Check sheet for the modelled part. Datum: model origin and axes. Units: mm. A direction names the side the tool comes from. Round coordinates to 2 decimals unless told otherwise and drop trailing zeros. Loops run counter-clockwise (first coordinate to the right, second up) from the corner with the lowest first, then second, coordinate; pieces in that order, holes last. Notation, with made-up numbers: (22.5, 40.5) -> (44.5, 40.5) arc R29 ccw to (44.5, 66.5) -> close; hole circle Ø5 at (-21, 70.25). An arc over 180 degrees is marked (long way). One line per question, with ' | ' between items.
```python
from build123d import *

# Parameters (mm, degrees)
SKETCH1_W           = 86.36
SKETCH1_H           = 50.8
SKETCH1_R           = 8.89
BOSS_EXTRUDE2_DEPTH = 25.4
CUT_EXTRUDE2_START  = 25.4
SKETCH1_3_R         = 13.97
SKETCH1_3_R_2       = 8.89
CUT_EXTRUDE2_DEPTH  = 5.08
CUT_EXTRUDE4_START  = -25.4
SKETCH1_4_R         = 13.97
SKETCH1_4_R_2       = 8.89
CUT_EXTRUDE4_DEPTH  = 5.08
SKETCH3_R           = 11.43
SKETCH3_R_2         = 5.55625
BOSS_EXTRUDE3_DEPTH = 10.16
SKETCH3_2_R         = 5.55625
CUT_EXTRUDE5_DEPTH  = 97.52
SKETCH4_W           = 66.04
SKETCH4_H           = 30.48
CUT_EXTRUDE6_DEPTH  = 51.8
BOSS_EXTRUDE4_START = 15.24
SKETCH5_R           = 17.78
SKETCH5_R_2         = 8.89
BOSS_EXTRUDE4_DEPTH = 5.08
BOSS_EXTRUDE5_START = -15.24
SKETCH5_2_R         = 17.78
SKETCH5_2_R_2       = 8.89
BOSS_EXTRUDE5_DEPTH = 5.08
FILLET1_R           = 2.54
FILLET2_R           = 2.54


with BuildPart() as part:
    # Sketch1 → Boss-Extrude2 (new body, symmetric)
    with BuildSketch(Plane.XY):
        Rectangle(SKETCH1_W, SKETCH1_H)
        Circle(SKETCH1_R, mode=Mode.SUBTRACT)
    extrude(amount=BOSS_EXTRUDE2_DEPTH, both=True)

    # Sketch1<3> → Cut-Extrude2 (cut)
    with BuildSketch(Plane.XY.offset(CUT_EXTRUDE2_START)):
        Circle(SKETCH1_3_R)
        Circle(SKETCH1_3_R_2, mode=Mode.SUBTRACT)
    extrude(amount=-CUT_EXTRUDE2_DEPTH, mode=Mode.SUBTRACT)

    # Sketch1<4> → Cut-Extrude4 (cut)
    with BuildSketch(Plane.XY.offset(CUT_EXTRUDE4_START)):
        Circle(SKETCH1_4_R)
        Circle(SKETCH1_4_R_2, mode=Mode.SUBTRACT)
    extrude(amount=CUT_EXTRUDE4_DEPTH, mode=Mode.SUBTRACT)

    # Sketch3 → Boss-Extrude3 (add)
    with BuildSketch(Plane(origin=(43.18, 0, 0), x_dir=(0, 0, -1), z_dir=(1, 0, 0))):
        Circle(SKETCH3_R)
        Circle(SKETCH3_R_2, mode=Mode.SUBTRACT)
    boss_extrude3 = extrude(amount=BOSS_EXTRUDE3_DEPTH)

    # Mirror1: Boss-Extrude3 across plane
    add(boss_extrude3.mirror(Plane(origin=(0, 0, 0), x_dir=(0, 0, 1), z_dir=(1, 0, 0))))

    # Sketch3<2> → Cut-Extrude5 (cut, through all)
    with BuildSketch(Plane(origin=(43.18, 0, 0), x_dir=(0, 0, -1), z_dir=(1, 0, 0))):
        Circle(SKETCH3_2_R)
    extrude(amount=-CUT_EXTRUDE5_DEPTH, mode=Mode.SUBTRACT)

    # Sketch4 → Cut-Extrude6 (cut, through all)
    with BuildSketch(Plane(origin=(0, 25.4, 0), x_dir=(1, 0, 0), z_dir=(0, 1, 0))):
        Rectangle(SKETCH4_W, SKETCH4_H)
    extrude(amount=-CUT_EXTRUDE6_DEPTH, mode=Mode.SUBTRACT)

    # Sketch5 → Boss-Extrude4 (add)
    with BuildSketch(Plane.XY.offset(BOSS_EXTRUDE4_START)):
        Circle(SKETCH5_R)
        Circle(SKETCH5_R_2, mode=Mode.SUBTRACT)
    extrude(amount=-BOSS_EXTRUDE4_DEPTH)

    # Sketch5<2> → Boss-Extrude5 (add)
    with BuildSketch(Plane.XY.offset(BOSS_EXTRUDE5_START)):
        Circle(SKETCH5_2_R)
        Circle(SKETCH5_2_R_2, mode=Mode.SUBTRACT)
    extrude(amount=BOSS_EXTRUDE5_DEPTH)

    # Fillet1
    fillet1_edges = [part.edges().sort_by_distance(p)[0] for p in [
        (-17.78, 0, 15.24),
        (-17.78, 0, -15.24),
    ]]
    fillet(fillet1_edges, radius=FILLET1_R)

    # Fillet2
    fillet2_edges = [part.edges().sort_by_distance(p)[0] for p in [
        (43.18, 0, 11.43),
        (-43.18, 0, 11.43),
    ]]
    fillet(fillet2_edges, radius=FILLET2_R)


solid = part.part
```
(1) Sectioned sample at A-A, the plane z = 0. Record the cut outline in (x, y).
Answer:
outline: (-53.34, -11.43) -> (-45.72, -11.43) arc R2.54 cw to (-43.18, -13.97) -> (-43.18, -25.4) -> (-33.02, -25.4) -> (-33.02, -5.56) -> (-53.34, -5.56) -> close; (-53.34, 5.56) -> (-33.02, 5.56) -> (-33.02, 25.4) -> (-43.18, 25.4) -> (-43.18, 13.97) arc R2.54 cw to (-45.72, 11.43) -> (-53.34, 11.43) -> close; (33.02, -25.4) -> (43.18, -25.4) -> (43.18, -13.97) arc R2.54 cw to (45.72, -11.43) -> (53.34, -11.43) -> (53.34, -5.56) -> (33.02, -5.56) -> close; (33.02, 5.56) -> (53.34, 5.56) -> (53.34, 11.43) -> (45.72, 11.43) arc R2.54 cw to (43.18, 13.97) -> (43.18, 25.4) -> (33.02, 25.4) -> close
(2) Go/stop test with flat-tipped pins: pin 1 (14 mm diameter, centred on x = 0.5, y = -4, fed in from -Z); pin 2 (1.5 mm diameter, centred on y = 9.5, z = -10.5, fed in from +X); pin 3 (5 mm diameter, centred on y = 14.5, z = 7, fed in from -X). Record where each tip stops, or that it passes through.
Answer:
pin 1: stops at z = -20.32 | pin 2: stops at x = 43.24 | pin 3: stops at x = -43.21
(3) Sectioned sample at C-C, the plane z = 21.5. Record the cut outline in (x, y).
Answer:
outline: (-43.18, -25.4) -> (43.18, -25.4) -> (43.18, 25.4) -> (-43.18, 25.4) -> close; hole circle Ø27.94 at (0, 0)
(4) Sectioned sample at B-B, the plane x = 29. Record the cut outline in (y, z), and give its area (3 significant figures).
Answer:
outline: (-25.4, -25.4) -> (25.4, -25.4) -> (25.4, -15.24) -> (-25.4, -15.24) -> close; (-25.4, 15.24) -> (25.4, 15.24) -> (25.4, 25.4) -> (-25.4, 25.4) -> close | area: 1,030 mm2
(5) Mould release check, pull along Z, two halves, no side actions. Record for faces 1 (the face through (-10, 12, -25.4)), 2 (the face through (-33.02, 6, 0)), 3 (the face through (-1.82, 13.85, -22.9)): +Z half, -Z half, draft (parallel to the pull), parting line (faces both ways), or undercut.
Answer:
face 1: -Z half | face 2: undercut | face 3: draft
(6) Scan lines: probe 1 along X at (y, z) = (13, -5.5); probe 2 along Z at (x, y) = (11.5, 11.5); probe 3 along Y at (x, z) = (0, 23). Record each from-to range of solid material in increasing order.
Answer:
probe 1: x = -43.18 to -33.02, 33.02 to 43.18 | probe 2: z = -25.4 to -10.16, 10.16 to 25.4 | probe 3: y = -25.4 to -13.97, 13.97 to 25.4
(7) Sectioned sample at D-D, the plane x = 0. Count the separate pieces of the cut face and the enclosed holes in it, and give its area (3 significant figures).
Answer:
separate pieces: 4 | enclosed holes: 0 | area: 754 mm2
(8) Set-up check for faces 4 (the face through (49.477, 3.433, -10.902)), 5 (the face through (33.02, 6, 0)), 6 (the face through (-0.2, -9.1, -20.32)), 7 (the face through (-43.18, 11, -11)), 8 (the face through (22, 0, 15.24)): record each of +Z, -Z, +X, -X, +Y, -Y from which the full face is reachable in a straight line by a thin tool's end or side.
Answer:
face 4: +X | face 5: +Y, -Y | face 6: -Z | face 7: -X | face 8: none
